Input: part model. Units: mm. Frame: model coordinates. A direction names the side the tool comes from. Coordinates: 2 decimals unless noted, no trailing zeros. Write each loop counter-clockwise with the first axis right and the second up, starting at its lowest first coordinate (ties: lowest second). Pieces come first, ordered by that corner, then holes. Notation, with made-up numbers: M 80.25,-4 L 120.25,-4 A21 ccw 120.25,16 Z; hole C -32.5,-9 d8. An arc over 180 degrees is marked long. Write each question's results on one line, items separated by ' | '. Start each with the question number.
1. Set-up query: faces 5 (the cylindrical face through (28.5, 14.8, 32.5)), 6 (the flat face through (12, 27, 158)), 7 (the flat face through (11, 0, 158)). Return all of +Z, -Z, +X, -X, +Y, -Y with unobstructed straight access to the full face (end or side cutting, diameter ignored); none if empty.
2. Section query D-D, the plane z = 270.5. Output: boundary loops of the cut face in (x, y), and give its area (3 significant figures).
3. Ray query, probe 1 along Y at (x, z) = (19.25, 297); probe 2 along X at (y, z) = (0.8, 265). Return the intervals inside material, ascending.
4. Section query A-A, the plane y = 15. Count the separate pieces of the cut face and the enclosed holes in it, and give its area (3 significant figures).
5. First-contact query: pin 1 (4 mm diameter, centred on x = 15, z = 300, fed in from -Y); pin 2 (6.5 mm diameter, centred on x = 15, z = 265, fed in from -Y). Flat tips, straight axial feed; report the tip coordinate or a pass-through.
6. Section query B-B, the plane x = 21.25. Output: boundary loops of the cut face in (y, z), and give its area (3 significant figures).
7. Section query C-C, the plane z = 184. Output: boundary loops of the cut face in (x, y), and give its area (3 significant figures).
8. Pull-direction query (X, two-part tool) for faces 1 (the cylindrical face through (1.5, 15.2, 197.5)), 2 (the flat face through (0, 5, 158)), 3 (the flat face through (27, 4, 158)), 4 (the flat face through (12, 3, 158)); classes: +X half, -X half, draft (parallel to the pull), parting line (faces both ways), or undercut.
```python
from build123d import *

# Parameters (mm, degrees)
SKETCH_1_W          = 30
SKETCH_1_H          = 30
SKETCH_1_W_2        = 24
SKETCH_1_H_2        = 24
EXTRUDE_1_DEPTH     = 320
SKETCH_2_R          = 10
CUT_EXTRUDE_1_DEPTH = 323.800247831
SKETCH_3_R          = 2.1
CUT_EXTRUDE_2_DEPTH = 323.800247831


with BuildPart() as part:
    # 草图1 → 拉伸-薄壁1 (new body)
    with BuildSketch(Plane.XY):
        with Locations((15, 15)):
            Rectangle(SKETCH_1_W, SKETCH_1_H)
        with Locations((15, 15)):
            Rectangle(SKETCH_1_W_2, SKETCH_1_H_2, mode=Mode.SUBTRACT)
    extrude(amount=EXTRUDE_1_DEPTH)

    # 草图2 → 切除-拉伸1 (cut, through all)
    with BuildSketch(Plane(origin=(30, 0, 0), x_dir=(0, 0, -1), z_dir=(1, 0, 0))):
        with Locations((-160, 15)):
            Circle(SKETCH_2_R)
        with BuildLine():
            Line((-277.5, 25), (-207.5, 25))
            ThreePointArc((-207.5, 25), (-197.5, 15), (-207.5, 5))
            Line((-207.5, 5), (-277.5, 5))
            ThreePointArc((-277.5, 5), (-287.5, 15), (-277.5, 25))
        make_face()
        with BuildLine():
            Line((-42.5, 25), (-112.5, 25))
            ThreePointArc((-112.5, 25), (-122.5, 15), (-112.5, 5))
            Line((-112.5, 5), (-42.5, 5))
            ThreePointArc((-42.5, 5), (-32.5, 15), (-42.5, 25))
        make_face()
    extrude(amount=-CUT_EXTRUDE_1_DEPTH, mode=Mode.SUBTRACT)

    # 草图3 → 切除-拉伸2 (cut, through all)
    with BuildSketch(Plane(origin=(0, 30, 0), x_dir=(1, 0, 0), z_dir=(0, 1, 0))):
        with Locations(Location((15, -20, 0), (0, 0, 270))):
            Circle(SKETCH_3_R)
        with Locations(Location((15, -55, 0), (0, 0, 270))):
            Circle(SKETCH_3_R)
        with Locations(Location((15, -90, 0), (0, 0, 270))):
            Circle(SKETCH_3_R)
        with Locations(Location((15, -125, 0), (0, 0, 270))):
            Circle(SKETCH_3_R)
        with Locations(Location((15, -300, 0), (0, 0, 90))):
            Circle(SKETCH_3_R)
        with Locations(Location((15, -265, 0), (0, 0, 90))):
            Circle(SKETCH_3_R)
        with Locations(Location((15, -230, 0), (0, 0, 90))):
            Circle(SKETCH_3_R)
        with Locations(Location((15, -195, 0), (0, 0, 90))):
            Circle(SKETCH_3_R)
        with Locations(Location((15, -160, 0), (0, 0, 270))):
            Circle(SKETCH_3_R)
    extrude(amount=-CUT_EXTRUDE_2_DEPTH, mode=Mode.SUBTRACT)


solid = part.part
```
Answer:
1) face 5: +X, -X | face 6: +Z, -Z | face 7: +Z, -Z, +X, -X, -Y
2) outline: M 0,0 L 30,0 L 30,5 L 27,5 L 27,3 L 3,3 L 3,5 L 0,5 Z; M 0,25 L 3,25 L 3,27 L 27,27 L 27,25 L 30,25 L 30,30 L 0,30 Z | area: 204 mm^2
3) probe 1: 0 to 3, 27 to 30 | probe 2: 0 to 12.9, 17.1 to 30
4) separate pieces: 8 | enclosed holes: 0 | area: 720 mm^2
5) pin 1: through | pin 2: y = 0
6) outline: M 0,0 L 3,0 L 3,320 L 0,320 Z; M 27,0 L 30,0 L 30,320 L 27,320 Z | area: 1,920 mm^2
7) outline: M 0,0 L 30,0 L 30,30 L 0,30 Z; hole M 3,3 L 27,3 L 27,27 L 3,27 Z | area: 324 mm^2
8) face 1: draft | face 2: -X half | face 3: undercut | face 4: undercut
